Geometry check sheet. Reference: the model listing, model coordinates, mm. A direction names the side the tool comes from. Coordinates: 2 decimals unless noted, no trailing zeros. Loops run counter-clockwise (first coordinate to the right, second up) from the corner with the lowest first, then second, coordinate; pieces in that order, holes last. Notation, with made-up numbers: (-40, 9.5) -> (10, 9.5) arc R12 ccw to (10, 16.5) -> close; hole circle Ø6 at (10.25, 58.5). An arc over 180 degrees is marked (long way). Answer as a JSON object with one key per item and string values.
from build123d import *

# Parameters (mm, degrees)
MAKERBEAMFIX_DEPTH                      = 35
SKETCH2_R                               = 1.5
MAKERBEAMFIXHOLE_DEPTH                  = 5
SKETCH3_W                               = 12
SKETCH3_H                               = 12
SKETCH3_R                               = 4.1
MAKERBEAMTOOLBIGHEXASCREWDRIVER_DEPTH   = 20
SKETCH4_W                               = 8
SKETCH4_H                               = 8
SKETCH4_R                               = 1.5
MAKERBEAMTOOLSMALLHEXASCREWDRIVER_DEPTH = 10
SIMPLESCREWDRIVER3MM_COUNT              = 2
SIMPLESCREWDRIVER3MM_PITCH              = 20
SKETCH5_W                               = 8
SKETCH5_H                               = 8
SKETCH5_R                               = 2
BOSS_EXTRUDE4_DEPTH                     = 10
FILLET1_R                               = 3


with BuildPart() as part:
    # Sketch1 → MakerBeamFix (new body, symmetric)
    with BuildSketch(Plane.XY):
        Polygon((-5, 0), (5, 0), (5, 3), (1.45, 3), (1.45, 4), (-1.45, 4), (-1.45, 3), (-5, 3), align=None)
    extrude(amount=MAKERBEAMFIX_DEPTH, both=True)

    # Sketch2 → MakerBeamFixHole (cut, through all)
    with BuildSketch(Plane(origin=(0, 0, 0), x_dir=(-1, 0, 0), z_dir=(0, -1, 0))):
        Circle(SKETCH2_R)
    extrude(amount=-MAKERBEAMFIXHOLE_DEPTH, mode=Mode.SUBTRACT)

    # Sketch3 → MakerBeamToolBigHexaScrewDriver (add)
    with BuildSketch(Plane.ZY.offset(5)):
        with Locations((-29, -6)):
            Rectangle(SKETCH3_W, SKETCH3_H)
        with Locations((-29, -6)):
            Circle(SKETCH3_R, mode=Mode.SUBTRACT)
    extrude(amount=-MAKERBEAMTOOLBIGHEXASCREWDRIVER_DEPTH)

    # Sketch4 → MakerBeamToolSmallHexaScrewDriver (add)
    with BuildSketch(Plane.ZY.offset(5)):
        with Locations((-10, -4)):
            Rectangle(SKETCH4_W, SKETCH4_H)
        with Locations((-10, -4)):
            Circle(SKETCH4_R, mode=Mode.SUBTRACT)
    makerbeamtoolsmallhexascrewdriver = extrude(amount=-MAKERBEAMTOOLSMALLHEXASCREWDRIVER_DEPTH)

    # SimpleScrewDriver3mm: MakerBeamToolSmallHexaScrewDriver ×2
    with Locations(*[(0, 0, i * SIMPLESCREWDRIVER3MM_PITCH) for i in range(1, SIMPLESCREWDRIVER3MM_COUNT)]):
        add(makerbeamtoolsmallhexascrewdriver)

    # Sketch5 → Boss-Extrude4 (add)
    with BuildSketch(Plane.ZY.offset(5)):
        with Locations((31, -4)):
            Rectangle(SKETCH5_W, SKETCH5_H)
        with Locations((31, -4)):
            Circle(SKETCH5_R, mode=Mode.SUBTRACT)
    extrude(amount=-BOSS_EXTRUDE4_DEPTH)

    # Fillet1
    fillet1_edges = [part.edges().sort_by_distance(p)[0] for p in [
        (0, 0, -23),
        (5, -12, -35),
        (5, -12, -23),
        (0, 0, -6),
        (0, -8, -6),
        (0, -8, -14),
        (0, 0, -14),
        (0, 0, 14),
        (0, -8, 14),
        (0, -8, 6),
        (0, 0, 6),
        (0, -8, 35),
        (0, -8, 27),
        (0, 0, 27),
    ]]
    fillet(fillet1_edges, radius=FILLET1_R)


solid = part.part
1. Section check C-C, the plane x = 10.25. Record the boundary of the cut face in (y, z).
Evaluation:
{"outline": "(-12, -32) arc R3 ccw to (-9, -35) -> (0, -35) -> (0, -23) -> (-9, -23) arc R3 ccw to (-12, -26) -> close; hole circle Ø8.2 at (-6, -29)"}
2. Section check A-A, the plane z = -10. Record the boundary of the cut face in (x, y), then the cut area to 3 significant figures.
Evaluation:
{"outline": "(-5, -8) -> (5, -8) -> (5, -5.5) -> (-5, -5.5) -> close; (-5, -2.5) -> (5, -2.5) -> (5, 3) -> (1.45, 3) -> (1.45, 4) -> (-1.45, 4) -> (-1.45, 3) -> (-5, 3) -> close", "area": "82.9 mm^2"}
3. Tool access check on faces 1 (the face through (0.07, -0.86, -5.1)), 2 (the face through (3, 3, 0)), 3 (the face through (-1.43, 1.97, -0.45)). Record the directions out of +Z, -Z, +X, -X, +Y, -Y that give a thin tool (end or side, any length) a straight path to the whole face; none if there is none.
Evaluation:
{"face 1": "+X, -X, -Y", "face 2": "+Z, -Z, +X, +Y", "face 3": "+Y, -Y"}
4. Depth check by flat-ended pin: P1, Ø5, axis at x = 0.5, z = 1, coming from the -Y side; P2, Ø2, axis at x = 7.5, z = -3, coming from the -Y side; P3, Ø6, axis at y = 1.5, z = 5, coming from the +X side; P4, Ø1.6, axis at x = -2, z = 31.5, coming from the -Y side. Enter the tip coordinate at first touch or a pass-through.
Evaluation:
{"P1": "stops at y = -0.04", "P2": "passes through", "P3": "stops at x = 5", "P4": "stops at y = -8"}
5. Mould release check, pull along Z, two halves, no side actions. Record for faces 4 (the face through (-1.2, 0, 1.4)), 5 (the face through (-5, -3, -8)), 6 (the face through (5, -4, -35)), 7 (the face through (-0.07, -3.93, -11.5)): released by +Z, released by -Z, zero draft, split by the parting line, or undercut.
Evaluation:
{"face 4": "undercut", "face 5": "zero draft", "face 6": "released by -Z", "face 7": "undercut"}
6. Thickness scan on probe 1 along Y at (x, z) = (-3.5, 24); probe 2 along Y at (x, z) = (-2, 31); probe 3 along Y at (x, z) = (8, -31). Record the ranges inside material, lowest first. Write a range as from..to.
Evaluation:
{"probe 1": "y = 0..3", "probe 2": "y = -8..-6, -2..3", "probe 3": "y = -12..-9.58, -2.42..0"}
7. Section check B-B, the plane x = 3.25. State how many separate pieces and enclosed holes the cut face has, then the cut area to 3 significant figures.
Evaluation:
{"separate pieces": "1", "enclosed holes": "4", "area": "463 mm^2"}
